Part model, mm, in its own coordinate system. A direction names the side the tool comes from. Give positions to 0.01 mm unless a question says otherwise; leave off trailing zeros. Order: outer loops, then holes, each group sorted by start corner. A loop starts at its lowest first (then second) coordinate and runs counter-clockwise, first axis right, second up. Notation, with made-up numbers: (9, 35.5) - (58, 35.5) arc R36 ccw to (58, 71.5) - close; hole circle Ø6 at (55, -11). An arc over 180 degrees is marked (long way). One line per item, written item: value.
```python
from build123d import *

# Parameters (mm, degrees)
BOSS_EXTRUDE1_DEPTH = 1.524


with BuildPart() as part:
    # Sketch1 → Boss-Extrude1 (new body)
    with BuildSketch(Plane.XY):
        with BuildLine():
            Line((1.507959842, 1.524), (1.507959842, 0))
            Line((1.507959842, 0), (3.052407177, 0))
            Line((3.052407177, 0), (3.052407177, -1.566256329))
            ThreePointArc((3.052407177, -1.566256329), (-6.301435783, -9.155076444), (-17.769362765, -12.838990069))
            ThreePointArc((-17.769362765, -12.838990069), (-20.072635935, -12.471877617), (-22.228452392, -11.581768494))
            ThreePointArc((-22.228452392, -11.581768494), (-13.1022498, -10.612386305), (-5.053668942, -6.202440528))
            ThreePointArc((-5.053668942, -6.202440528), (-3.071218913, -3.363942956), (-2.252033724, 0))
            Line((-2.252033724, 0), (-2.252033724, 1.524))
            Line((-2.252033724, 1.524), (1.507959842, 1.524))
        make_face()
    extrude(amount=BOSS_EXTRUDE1_DEPTH)


solid = part.part
```
1) Cut at C-C, the plane x = -19. Give the cut face in (y, z).
Outcome:
outline: (-12.71, 0) - (-11.66, 0) - (-11.66, 1.52) - (-12.71, 1.52) - close
2) Pin check, flat tip, straight feed: pin 1 (0.8 mm diameter, centred on x = 2, z = 1, fed in from +Y). Stop position of the tip, or through.
Outcome:
pin 1: stops at y = 0
3) Which spindle directions (+Z, -Z, +X, -X, +Y, -Y) get a long thin tool onto all of the face, cutting with end or side? Do faces 1 (the flat face through (-4, -6, 1.524)), 2 (the flat face through (1.508, 1, 1)), 3 (the flat face through (-2.252, 1, 1)). Say none if no direction does.
Outcome:
face 1: +Z, +X, -X, +Y, -Y
face 2: +Z, -Z, +X, +Y
face 3: +Z, -Z, -X, +Y
4) Drill centre lines: line 1 along Y through (x, z) = (-15.5, 0.5); line 2 along Y through (x, z) = (-17.5, 0.8); line 3 along X through (y, z) = (-1.5, 1.1). Where is each one in solid material? Low to high. Write a range as from..to.
Outcome:
line 1: y = -12.47..-11.23
line 2: y = -12.8..-11.54
line 3: x = -2.45..3.05
5) Cut at B-B, the plane y = -3.25. Give the cut face in (x, z), then the cut area to 3 significant figures.
Outcome:
outline: (-3.02, 0) - (1.52, 0) - (1.52, 1.52) - (-3.02, 1.52) - close
area: 6.92 mm^2
6) Cut at A-A, the plane z = 0.7. Give the cut face in (x, y).
Outcome:
outline: (-22.23, -11.58) arc R10.01 ccw to (-17.77, -12.84) arc R32.67 ccw to (3.05, -1.57) - (3.05, 0) - (1.51, 0) - (1.51, 1.52) - (-2.25, 1.52) - (-2.25, 0) arc R9.39 cw to (-5.05, -6.2) arc R23.36 cw to start
